```python
from build123d import *

# Parameters (mm, degrees)
SKETCH1_R                                           = 23
SKETCH1_R_2                                         = 8
SKETCH1_R_3                                         = 3.5
BOSS_EXTRUDE1_DEPTH                                 = 5
SKETCH1_3_R                                         = 8
BOSS_EXTRUDE2_DEPTH                                 = 32
SKETCH2_R                                           = 2.5
CUT_EXTRUDE1_DEPTH                                  = 37
CHAMFER2_SIZE                                       = 0.5
CSK_FOR_M6_COUNTERSUNK_FLAT_HEAD_SCREW2_D           = 7
CSK_FOR_M6_COUNTERSUNK_FLAT_HEAD_SCREW2_DEPTH       = 5
CSK_FOR_M6_COUNTERSUNK_FLAT_HEAD_SCREW2_CSINK_D     = 9
CSK_FOR_M6_COUNTERSUNK_FLAT_HEAD_SCREW2_CSINK_ANGLE = 90
CSK_FOR_M6_COUNTERSUNK_FLAT_HEAD_SCREW2_TIP         = 2.103012167


with BuildPart() as part:
    # Sketch1 → Boss-Extrude1 (new body)
    with BuildSketch(Plane.XY):
        Circle(SKETCH1_R)
        Circle(SKETCH1_R_2, mode=Mode.SUBTRACT)
        with Locations((0, 15)):
            Circle(SKETCH1_R_3, mode=Mode.SUBTRACT)
    extrude(amount=BOSS_EXTRUDE1_DEPTH)

    # Sketch1<3> → Boss-Extrude2 (add)
    with BuildSketch(Plane.XY):
        Circle(SKETCH1_3_R)
    extrude(amount=BOSS_EXTRUDE2_DEPTH)

    # Sketch2 → Cut-Extrude1 (cut)
    with BuildSketch(Plane.XY.offset(32)):
        Circle(SKETCH2_R)
    extrude(amount=-CUT_EXTRUDE1_DEPTH, mode=Mode.SUBTRACT)

    # Chamfer2
    chamfer2_edges = [part.edges().sort_by_distance(p)[0] for p in [
        (-8, 0, 32),
        (-23, 0, 0),
        (-2.5, 0, 32),
        (-23, 0, 5),
    ]]
    chamfer(chamfer2_edges, length=CHAMFER2_SIZE)

    # CSK for M6 Countersunk Flat Head Screw2
    with Locations(Plane(origin=(0, 0, 0), x_dir=(-1, 0, 0), z_dir=(0, 0, -1))):
        with Locations((0, 15)):
            CounterSinkHole(CSK_FOR_M6_COUNTERSUNK_FLAT_HEAD_SCREW2_D / 2, CSK_FOR_M6_COUNTERSUNK_FLAT_HEAD_SCREW2_CSINK_D / 2, depth=CSK_FOR_M6_COUNTERSUNK_FLAT_HEAD_SCREW2_DEPTH, counter_sink_angle=CSK_FOR_M6_COUNTERSUNK_FLAT_HEAD_SCREW2_CSINK_ANGLE)
            with Locations((0, 0, -(CSK_FOR_M6_COUNTERSUNK_FLAT_HEAD_SCREW2_DEPTH + CSK_FOR_M6_COUNTERSUNK_FLAT_HEAD_SCREW2_TIP / 2))):  # 118° drill point
                Cone(0, CSK_FOR_M6_COUNTERSUNK_FLAT_HEAD_SCREW2_D / 2, CSK_FOR_M6_COUNTERSUNK_FLAT_HEAD_SCREW2_TIP, mode=Mode.SUBTRACT)


solid = part.part
```
Geometry: final body of the model. Coordinates: model frame, mm. A direction names the side the tool comes from. Give positions to 0.01 mm unless a question says otherwise; leave off trailing zeros. Order: outer loops, then holes, each group sorted by start corner. A loop starts at its lowest first (then second) coordinate and runs counter-clockwise, first axis right, second up. Notation, with made-up numbers: M 22.25,-39 L 29.25,-39 A28 ccw 29.25,-14 Z; hole C 61.25,52.25 d5. An arc over 180 degrees is marked long. Answer as CSV lines item,"result". Start each with the question number.
1) Cut plane D-D (z = 3). Output: boundary loops of the cut face in (x, y), then the cut area to 3 significant figures.
2) Cut plane C-C (z = 29). Output: boundary loops of the cut face in (x, y), then the cut area to 3 significant figures.
3) Cut plane B-B (x = 0). Output: boundary loops of the cut face in (y, z).
4) First-contact query: P1, Ø12, axis at y = -15, z = 18.5, coming from the -X side; P2, Ø10, axis at x = -7, z = 8, coming from the +Y side; P3, Ø8, axis at y = -18, z = 5, coming from the +X side; P4, Ø1.5, axis at x = 18, y = 12.5, coming from the +Z side. Flat tips, straight axial feed; report the tip coordinate or a pass-through.
5) Mould query, pull axis X, two halves, no side actions, for faces 3 (the cylindrical face through (-2.994, 22.804, 2.472)), 4 (the cylindrical face through (-0.759, 11.583, 2.972)), 5 (the flat face through (0, -10, 5)). Classes: +X half, -X half, draft (parallel to the pull), parting line (faces both ways), or undercut.
6) Cut plane A-A (y = 0). Output: boundary loops of the cut face in (x, z), then the cut area to 3 significant figures.
7) Set-up query: faces 1 (the cylindrical face through (-0.54, -2.44, 15.97)), 2 (the cylindrical face through (-1.73, -7.81, 18.06)). Return all of +Z, -Z, +X, -X, +Y, -Y with unobstructed straight access to the full face (end or side cutting, diameter ignored); none if empty.
8) Line query: line 1 (Y direction, x = 0, z = 3); line 2 (Y direction, x = 0, z = 21.5); line 3 (Z direction, x = 15.5, y = 11.5). Output: solid intervals per line, ascending. Write a range as from..to.
Findings below:
1,outline,"C 0,0 d46; hole C 0,15 d7; hole C 0,0 d5"
1,area,"1,600 mm²"
2,outline,"C 0,0 d16; hole C 0,0 d5"
2,area,"181 mm²"
3,outline,"M -23,0.5 L -22.5,0 L -2.5,0 L -2.5,31.5 L -3,32 L -7.5,32 L -8,31.5 L -8,5 L -22.5,5 L -23,4.5 Z; M 2.5,0 L 10.5,0 L 11.5,1 L 11.5,5 L 8,5 L 8,31.5 L 7.5,32 L 3,32 L 2.5,31.5 Z; M 18.5,1 L 19.5,0 L 22.5,0 L 23,0.5 L 23,4.5 L 22.5,5 L 18.5,5 Z"
4,P1,"passes through"
4,P2,"stops at y = 22.74"
4,P3,"stops at x = 18.22"
4,P4,"stops at z = 5"
5,face 3,"parting line"
5,face 4,"undercut"
5,face 5,"draft"
6,outline,"M -23,0.5 L -22.5,0 L -2.5,0 L -2.5,31.5 L -3,32 L -7.5,32 L -8,31.5 L -8,5 L -22.5,5 L -23,4.5 Z; M 2.5,0 L 22.5,0 L 23,0.5 L 23,4.5 L 22.5,5 L 8,5 L 8,31.5 L 7.5,32 L 3,32 L 2.5,31.5 Z"
6,area,"501 mm²"
7,face 1,"+Z, -Z"
7,face 2,"+Z"
8,line 1,"y = -23..-2.5, 2.5..11.5, 18.5..23"
8,line 2,"y = -8..-2.5, 2.5..8"
8,line 3,"z = 0..5"
